Could you check a few things on this model? Use its own coordinates, in mm. A direction names the side the tool comes from. Give positions to 0.01 mm unless a question says otherwise; leave off trailing zeros. Order: outer loops, then holes, each group sorted by start corner. A loop starts at its lowest first (then second) coordinate and runs counter-clockwise, first axis right, second up. Notation, with made-up numbers: (13.5, 34.25) - (20.5, 34.25) arc R25 ccw to (20.5, 52.25) - close; hole circle Ø9 at (18, -26). An arc over 180 degrees is marked (long way). Put each result on its own line as item: value.
from build123d import *

# Parameters (mm, degrees)
BOSS_EXTRUDE1_DEPTH     = 35
SKETCH4_3_R             = 1.6
BOSS_EXTRUDE2_DEPTH     = 10
SKETCH6_R               = 3.6
BOSS_EXTRUDE4_DEPTH     = 5
CUT_EXTRUDE3_DEPTH      = 198.693522892
CUT_EXTRUDE3_DEPTH_BACK = 198.693522892
SKETCH10_R              = 1.6
CUT_EXTRUDE4_REACH      = 212.71
SKETCH11_W              = 8.5
SKETCH11_H              = 21.5
SKETCH12_W              = 12.5
SKETCH12_H              = 2
CUT_EXTRUDE5_DEPTH      = 6
SKETCH13_W              = 6
SKETCH13_H              = 7.2
CUT_EXTRUDE6_DEPTH      = 15
SKETCH14_W              = 6
SKETCH14_H              = 7.2
CUT_EXTRUDE7_DEPTH      = 15


with BuildPart() as part:
    # Sketch4 → Boss-Extrude1 (new body)
    with BuildSketch(Plane.XY):
        with BuildLine():
            Line((43.355273195, 152.732885516), (43.387199595, 166.493163991))
            ThreePointArc((43.387199595, 166.493163991), (40.904598686, 172.516316495), (34.887222474, 175.012885516))
            Line((34.887222474, 175.012885516), (-15.022777526, 175.012885516))
            ThreePointArc((-15.022777526, 175.012885516), (-21.033185166, 172.523293156), (-23.522777526, 166.512885516))
            Line((-23.522777526, 166.512885516), (-23.522777526, 71.512885516))
            ThreePointArc((-23.522777526, 71.512885516), (-21.033185166, 65.502477876), (-15.022777526, 63.012885516))
            Line((-15.022777526, 63.012885516), (79.977222474, 63.012885516))
            ThreePointArc((79.977222474, 63.012885516), (85.987630114, 65.502477876), (88.477222474, 71.512885516))
            Line((88.477222474, 71.512885516), (88.477222474, 144.232885516))
            ThreePointArc((88.477222474, 144.232885516), (85.987630114, 150.243293156), (79.977222474, 152.732885516))
            Line((79.977222474, 152.732885516), (77.987222474, 152.732885516))
            Line((77.987222474, 152.732885516), (71.637222474, 152.732885516))
            Line((71.637222474, 152.732885516), (50.047222474, 152.732885516))
            Line((50.047222474, 152.732885516), (43.697222474, 152.732885516))
            Line((43.697222474, 152.732885516), (43.355273195, 152.732885516))
        make_face()
        with BuildLine():
            ThreePointArc((37.387215745, 166.507085068), (36.657039007, 168.27860051), (34.887222474, 169.012885516))
            Line((34.887222474, 169.012885516), (-15.022777526, 169.012885516))
            ThreePointArc((-15.022777526, 169.012885516), (-16.790544479, 168.280652469), (-17.522777526, 166.512885516))
            Line((-17.522777526, 166.512885516), (-17.522777526, 71.512885516))
            ThreePointArc((-17.522777526, 71.512885516), (-16.790544479, 69.745118563), (-15.022777526, 69.012885516))
            Line((-15.022777526, 69.012885516), (79.977222474, 69.012885516))
            ThreePointArc((79.977222474, 69.012885516), (81.744989427, 69.745118563), (82.477222474, 71.512885516))
            Line((82.477222474, 71.512885516), (82.477222474, 144.232885516))
            ThreePointArc((82.477222474, 144.232885516), (81.744989427, 146.000652469), (79.977222474, 146.732885516))
            Line((79.977222474, 146.732885516), (77.987222474, 146.732885516))
            Line((77.987222474, 146.732885516), (71.637222474, 146.732885516))
            Line((71.637222474, 146.732885516), (50.047222474, 146.732885516))
            Line((50.047222474, 146.732885516), (43.697222474, 146.732885516))
            Line((43.697222474, 146.732885516), (39.887222474, 146.732885516))
            ThreePointArc((39.887222474, 146.732885516), (38.091175602, 147.476836668), (37.347229203, 149.272885508))
            Line((37.347229203, 149.272885508), (37.387215745, 166.507085068))
        make_face(mode=Mode.SUBTRACT)
    extrude(amount=BOSS_EXTRUDE1_DEPTH)

    # Sketch4<3> → Boss-Extrude2 (add)
    with BuildSketch(Plane.XY):
        with BuildLine():
            Line((37.347229203, 149.272885508), (37.387215745, 166.507085068))
            ThreePointArc((37.387215745, 166.507085068), (36.657039007, 168.27860051), (34.887222474, 169.012885516))
            Line((34.887222474, 169.012885516), (-15.022777526, 169.012885516))
            ThreePointArc((-15.022777526, 169.012885516), (-16.790544479, 168.280652469), (-17.522777526, 166.512885516))
            Line((-17.522777526, 166.512885516), (-17.522777526, 71.512885516))
            ThreePointArc((-17.522777526, 71.512885516), (-16.790544479, 69.745118563), (-15.022777526, 69.012885516))
            Line((-15.022777526, 69.012885516), (79.977222474, 69.012885516))
            ThreePointArc((79.977222474, 69.012885516), (81.744989427, 69.745118563), (82.477222474, 71.512885516))
            Line((82.477222474, 71.512885516), (82.477222474, 144.232885516))
            ThreePointArc((82.477222474, 144.232885516), (81.744989427, 146.000652469), (79.977222474, 146.732885516))
            Line((79.977222474, 146.732885516), (77.987222474, 146.732885516))
            Line((77.987222474, 146.732885516), (71.637222474, 146.732885516))
            Line((71.637222474, 146.732885516), (50.047222474, 146.732885516))
            Line((50.047222474, 146.732885516), (43.697222474, 146.732885516))
            Line((43.697222474, 146.732885516), (39.887222474, 146.732885516))
            ThreePointArc((39.887222474, 146.732885516), (38.091175602, 147.476836668), (37.347229203, 149.272885508))
        make_face()
        with Locations((-7.822777526, 160.912885516)):
            Circle(SKETCH4_3_R, mode=Mode.SUBTRACT)
        with Locations((31.877222474, 160.912885516)):
            Circle(SKETCH4_3_R, mode=Mode.SUBTRACT)
        with Locations((68.877222474, 74.812885516)):
            Circle(SKETCH4_3_R, mode=Mode.SUBTRACT)
        with Locations((-12.522777526, 74.012885516)):
            Circle(SKETCH4_3_R, mode=Mode.SUBTRACT)
    extrude(amount=BOSS_EXTRUDE2_DEPTH)

    # Sketch6 → Boss-Extrude4 (add)
    with BuildSketch(Plane.XY.offset(10)):
        with Locations((68.877222474, 74.812885516)):
            Circle(SKETCH6_R)
        with Locations((-12.522777526, 74.012885516)):
            Circle(SKETCH6_R)
        with Locations((31.877222474, 160.912885516)):
            Circle(SKETCH6_R)
        with Locations((-7.822777526, 160.912885516)):
            Circle(SKETCH6_R)
    extrude(amount=BOSS_EXTRUDE4_DEPTH)

    # Sketch10 → Cut-Extrude3 (cut, two sides: drawn at the far end of the back side and taken through both)
    with BuildSketch(Plane.XY.offset(10).offset(-CUT_EXTRUDE3_DEPTH_BACK)):
        with Locations((-7.822777526, 160.912885516)):
            Circle(SKETCH10_R)
        with Locations((-12.522777526, 74.012885516)):
            Circle(SKETCH10_R)
        with Locations((31.877222474, 160.912885516)):
            Circle(SKETCH10_R)
        with Locations((68.877222474, 74.812885516)):
            Circle(SKETCH10_R)
    extrude(amount=CUT_EXTRUDE3_DEPTH + CUT_EXTRUDE3_DEPTH_BACK, mode=Mode.SUBTRACT)

    # Sketch11 → Cut-Extrude4 (cut, up to next)
    with BuildSketch(Plane(origin=(88.477222474, 0, 0), x_dir=(0, 0, -1), z_dir=(1, 0, 0)), mode=Mode.PRIVATE) as cut_extrude4_sk1:
        with Locations((-20.242185592, 81.762885516)):
            Rectangle(SKETCH11_W, SKETCH11_H)
    cut_extrude4_tool1 = extrude(cut_extrude4_sk1.sketch, amount=-CUT_EXTRUDE4_REACH, mode=Mode.PRIVATE) & part.part
    add(cut_extrude4_tool1.solids().sort_by_distance((88.477222, 81.762886, 20.242186))[0], mode=Mode.SUBTRACT)

    # Sketch12 → Cut-Extrude5 (cut)
    with BuildSketch(Plane(origin=(0, 175.012885516, 0), x_dir=(1, 0, 0), z_dir=(0, 1, 0))):
        with Locations((15.887215745, -17)):
            Rectangle(SKETCH12_W, SKETCH12_H)
    extrude(amount=-CUT_EXTRUDE5_DEPTH, mode=Mode.SUBTRACT)

    # Sketch13 → Cut-Extrude6 (cut)
    with BuildSketch(Plane.XY.offset(35)):
        with Locations((85.477222474, 140.332885516)):
            Rectangle(SKETCH13_W, SKETCH13_H)
        with Locations((85.477222474, 119.332885516)):
            Rectangle(SKETCH13_W, SKETCH13_H)
        with Locations((85.477222474, 99.332885516)):
            Rectangle(SKETCH13_W, SKETCH13_H)
    extrude(amount=-CUT_EXTRUDE6_DEPTH, mode=Mode.SUBTRACT)

    # Sketch14 → Cut-Extrude7 (cut)
    with BuildSketch(Plane.XY.offset(35)):
        with Locations((-20.522777526, 101.112885516)):
            Rectangle(SKETCH14_W, SKETCH14_H)
        with Locations((-20.522777526, 137.812885516)):
            Rectangle(SKETCH14_W, SKETCH14_H)
    extrude(amount=-CUT_EXTRUDE7_DEPTH, mode=Mode.SUBTRACT)


solid = part.part
1) If I drill on line 1 (X direction, y = 156, z = 12.5); line 2 (Y direction, x = 64, z = 19); line 3 (Y direction, x = 4, z = 23), over which ranges is the centre line in solid material (lowest first)? Write a range as [from, to].
Filled in:
line 1: x = [-23.52, -17.52], [37.36, 43.36]
line 2: y = [63.01, 69.01], [146.73, 152.73]
line 3: y = [63.01, 69.01], [169.01, 175.01]
2) I'm going to push flat-ended pins straight in: pin 1 (2.5 mm diameter, centred on x = 68.88, y = 74.81, fed in from -Z); pin 2 (1.8 mm diameter, centred on x = -22, z = 24, fed in from +Y); pin 3 (4 mm diameter, centred on y = 163, z = 21, fed in from +X); pin 4 (6 mm diameter, centred on x = 58, y = 155.5, fed in from -Z). Where does each tip first touch, or does it pass through?
Filled in:
pin 1: passes through
pin 2: stops at y = 172.46
pin 3: stops at x = 43.38
pin 4: stops at z = 0
3) Which directions (+Z, -Z, +X, -X, +Y, -Y) give clear straight access to the entire face, cutting with the end or side of a thin tool? Please do faces 4 (the flat face through (85, 119, 20)), 5 (the flat face through (82.477, 107, 22)), 6 (the flat face through (85, 82, 24.492)).
Filled in:
face 4: +Z, +X
face 5: +Z
face 6: +X
4) Suppose I cut it at A-A, the plane y = 81.5. List the corners of the cut face in (x, z) for me, and give its area (3 significant figures).
Filled in:
outline: (-23.52, 0) - (88.48, 0) - (88.48, 15.99) - (82.48, 15.99) - (82.48, 10) - (-17.52, 10) - (-17.52, 35) - (-23.52, 35) - close; (82.48, 24.49) - (88.48, 24.49) - (88.48, 35) - (82.48, 35) - close
area: 1,370 mm^2
5) Suppose I cut it at D-D, the plane y = 101.5. List the corners of the cut face in (x, z) for me, and give its area (3 significant figures).
Filled in:
outline: (-23.52, 0) - (88.48, 0) - (88.48, 20) - (82.48, 20) - (82.48, 10) - (-17.52, 10) - (-17.52, 20) - (-23.52, 20) - close
area: 1,240 mm^2
6) Suppose I cut it at B-B, the plane z = 11.5. State how many separate pieces and enclosed holes the cut face has, and give its area (3 significant figures).
Filled in:
separate pieces: 5
enclosed holes: 5
area: 2,600 mm^2
7) We'd pull the mould along X, two halves only. Please class faces 1 (the flat face through (85, 140, 20)), 2 (the cylindrical face through (31.53, 159.35, 7.4)), 3 (the cylindrical face through (-20.967, 172.589, 17.255)): pulls with the +X half, pulls with the -X half, needs draft (parallel to the pull), parting line crosses it, or undercut.
Filled in:
face 1: needs draft
face 2: undercut
face 3: pulls with the -X half
8) Suppose I cut it at C-C, the plane x = 57. List the corners of the cut face in (y, z) for me, and give its area (3 significant figures).
Filled in:
outline: (63.01, 0) - (152.73, 0) - (152.73, 35) - (146.73, 35) - (146.73, 10) - (69.01, 10) - (69.01, 35) - (63.01, 35) - close
area: 1,200 mm^2
